from build123d import *

# Parameters (mm, degrees)
SKETCH_1_W               = 145
SKETCH_1_H               = 141.74
EXTRUDE_1_DEPTH          = 1
FILLET_1_R               = 15
EXTRUDE_2_DEPTH          = 1
SKETCH_3_R               = 2.5
SKETCH_3_R_2             = 1.5
CUT_EXTRUDE_1_DEPTH      = 127.962285976
PATTERN_CIRCULAR_1_COUNT = 4
CUT_EXTRUDE_2_DEPTH      = 127.962285976
FILLET_2_R               = 15
FILLET_3_R               = 3
CUT_EXTRUDE_3_DEPTH      = 121.297119251
SKETCH_6_W               = 36
SKETCH_6_H               = 1
EXTRUDE_3_DEPTH          = 6
FILLET_4_R               = 10
FILLET_5_R               = 1.5
SKETCH_8_W               = 20
SKETCH_8_H               = 8
SKETCH_8_R               = 1.5
EXTRUDE_5_DEPTH          = 1
FILLET_8_R               = 3
FILLET_9_R               = 5


with BuildPart() as part:
    # 草图1 → 凸台-拉伸1 (new body)
    with BuildSketch(Plane(origin=(0, 0, 0), x_dir=(1, 0, 0), z_dir=(0, 1, 0))):
        Rectangle(SKETCH_1_W, SKETCH_1_H)
    extrude(amount=EXTRUDE_1_DEPTH)

    # 圆角1
    fillet_1_edges = [part.edges().sort_by_distance(p)[0] for p in [
        (-72.5, 0.5, -70.87),
    ]]
    fillet(fillet_1_edges, radius=FILLET_1_R)

    # 草图2 → 凸台-拉伸2 (add)
    with BuildSketch(Plane(origin=(0, 1, 0), x_dir=(1, 0, 0), z_dir=(0, 1, 0))):
        with BuildLine():
            Line((-92.747934341, -37.981190359), (-72.5, -22.981190359))
            Line((-72.5, -22.981190359), (-72.5, -81.673631364))
            Line((-72.5, -81.673631364), (-94.803937304, -53.673631364))
            ThreePointArc((-94.803937304, -53.673631364), (-97.10678595, -45.391007263), (-92.747934341, -37.981190359))
        make_face()
    extrude(amount=-EXTRUDE_2_DEPTH)

    # 草图3 → 切除-拉伸1 (cut, through all)
    with BuildSketch(Plane(origin=(0, 1, 0), x_dir=(1, 0, 0), z_dir=(0, 1, 0))):
        with Locations(Location((-86.2, -46.82, 0), (0, 0, 270))):
            Circle(SKETCH_3_R)
        with Locations(Location((-93.2, -46.82, 0), (0, 0, 270))):
            Circle(SKETCH_3_R_2)
    cut_extrude_1 = extrude(amount=-CUT_EXTRUDE_1_DEPTH, mode=Mode.SUBTRACT)

    # 阵列(圆周)1: 切除-拉伸1 ×4 about axis
    pattern_circular_1_axis = Axis((-86.2, 0, 46.82), (0, 1, 0))
    for i in range(1, PATTERN_CIRCULAR_1_COUNT):
        add(cut_extrude_1.rotate(pattern_circular_1_axis, i * 360 / PATTERN_CIRCULAR_1_COUNT), mode=Mode.SUBTRACT)

    # 草图4 → 切除-拉伸2 (cut, through all)
    with BuildSketch(Plane(origin=(0, 1, 0), x_dir=(1, 0, 0), z_dir=(0, 1, 0))):
        Polygon((-72.5, -70.87), (-94.803937304, -53.673631364), (-72.5, -88.862813476), align=None)
    extrude(amount=-CUT_EXTRUDE_2_DEPTH, mode=Mode.SUBTRACT)

    # 圆角2
    fillet_2_edges = [part.edges().sort_by_distance(p)[0] for p in [
        (-72.5, 0.5, 70.87),
    ]]
    fillet(fillet_2_edges, radius=FILLET_2_R)

    # 圆角3
    fillet_3_edges = [part.edges().sort_by_distance(p)[0] for p in [
        (-72.5, 0.5, 22.981190359),
    ]]
    fillet(fillet_3_edges, radius=FILLET_3_R)

    # 草图5 → 切除-拉伸3 (cut, through all)
    with BuildSketch(Plane(origin=(0, 1, 0), x_dir=(1, 0, 0), z_dir=(0, 1, 0))):
        with BuildLine():
            Line((-50, 60.87), (50, 60.87))
            ThreePointArc((50, 60.87), (58, 52.87), (50, 44.87))
            Line((50, 44.87), (-50, 44.87))
            ThreePointArc((-50, 44.87), (-58, 52.87), (-50, 60.87))
        make_face()
        with BuildLine():
            Line((-50, 39.87), (50, 39.87))
            ThreePointArc((50, 39.87), (58, 31.87), (50, 23.87))
            Line((50, 23.87), (-50, 23.87))
            ThreePointArc((-50, 23.87), (-58, 31.87), (-50, 39.87))
        make_face()
        with BuildLine():
            Line((-50, 18.87), (50, 18.87))
            ThreePointArc((50, 18.87), (58, 10.87), (50, 2.87))
            Line((50, 2.87), (-50, 2.87))
            ThreePointArc((-50, 2.87), (-58, 10.87), (-50, 18.87))
        make_face()
        with BuildLine():
            Line((-50, -2.13), (50, -2.13))
            ThreePointArc((50, -2.13), (58, -10.13), (50, -18.13))
            Line((50, -18.13), (-50, -18.13))
            ThreePointArc((-50, -18.13), (-58, -10.13), (-50, -2.13))
        make_face()
        with BuildLine():
            Line((-50, -23.13), (50, -23.13))
            ThreePointArc((50, -23.13), (58, -31.13), (50, -39.13))
            Line((50, -39.13), (-50, -39.13))
            ThreePointArc((-50, -39.13), (-58, -31.13), (-50, -23.13))
        make_face()
        with BuildLine():
            Line((-50, -44.13), (50, -44.13))
            ThreePointArc((50, -44.13), (58, -52.13), (50, -60.13))
            Line((50, -60.13), (-50, -60.13))
            ThreePointArc((-50, -60.13), (-58, -52.13), (-50, -44.13))
        make_face()
    extrude(amount=-CUT_EXTRUDE_3_DEPTH, mode=Mode.SUBTRACT)

    # 草图6 → 凸台-拉伸3 (add)
    with BuildSketch(Plane(origin=(0, 0, -70.87), x_dir=(-1, 0, 0), z_dir=(0, 0, -1))):
        with Locations((-54.5, 0.5)):
            Rectangle(SKETCH_6_W, SKETCH_6_H)
    extrude(amount=EXTRUDE_3_DEPTH)

    # 圆角4
    fillet_4_edges = [part.edges().sort_by_distance(p)[0] for p in [
        (72.5, 0.5, -76.87),
    ]]
    fillet(fillet_4_edges, radius=FILLET_4_R)

    # 圆角5
    fillet_5_edges = [part.edges().sort_by_distance(p)[0] for p in [
        (36.5, 0.5, -76.87),
    ]]
    fillet(fillet_5_edges, radius=FILLET_5_R)

    # 草图8 → 凸台-拉伸5 (add)
    with BuildSketch(Plane(origin=(0, 1, 0), x_dir=(1, 0, 0), z_dir=(0, 1, 0))):
        with Locations((52.5, -74.87)):
            Rectangle(SKETCH_8_W, SKETCH_8_H)
        with Locations(Location((47.504832843, -73.37, 0), (0, 0, 270))):
            Circle(SKETCH_8_R, mode=Mode.SUBTRACT)
        with Locations(Location((57.504832843, -73.37, 0), (0, 0, 270))):
            Circle(SKETCH_8_R, mode=Mode.SUBTRACT)
    extrude(amount=-EXTRUDE_5_DEPTH)

    # 圆角8
    fillet_8_edges = [part.edges().sort_by_distance(p)[0] for p in [
        (62.5, 0.5, 70.87),
        (62.5, 0.5, 78.87),
        (42.5, 0.5, 78.87),
        (42.5, 0.5, 70.87),
    ]]
    fillet(fillet_8_edges, radius=FILLET_8_R)

    # 圆角9
    fillet_9_edges = [part.edges().sort_by_distance(p)[0] for p in [
        (72.5, 0.5, 70.87),
    ]]
    fillet(fillet_9_edges, radius=FILLET_9_R)


solid = part.part
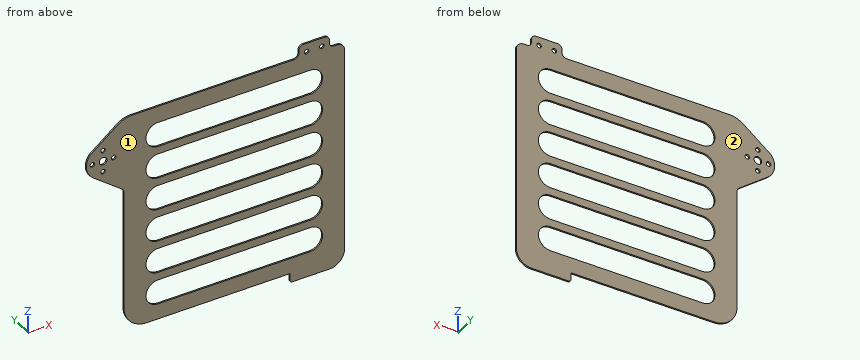
Verification items for the finished model (mm, model axes). Face numbers are marked on the shaded views. Coordinates: 2 decimals unless noted, no trailing zeros. Order: outer loops, then holes, each group sorted by start corner. A loop starts at its lowest first (then second) coordinate and runs counter-clockwise, first axis right, second up.
Item 1: Section check C-C, the plane y = 0.65. Give the number of separate pieces and of enclosed holes in the cut face, then the cut area to 3 significant figures.
Filled in:
separate pieces: 1
enclosed holes: 13
area: 10,700 mm2
Item 2: Depth check by flat-ended pin: pin 1 (6 mm diameter, centred on x = -62.5, z = 62.5, fed in from -Y); pin 2 (0.5 mm diameter, centred on x = 6.5, y = 0.5, fed in from -Z); pin 3 (4.5 mm diameter, centred on x = -86.2, z = 46.82, fed in from +Y); pin 4 (0.5 mm diameter, centred on x = 3, y = 0.5, fed in from +Z). Enter the tip coordinate at first touch or a pass-through.
Filled in:
pin 1: stops at y = 0
pin 2: stops at z = -70.87
pin 3: passes through
pin 4: stops at z = 70.87
Item 3: Section check A-A, the plane z = -52.87. Enter the section's corners in (x, y), then the cut area to 3 significant figures.
Filled in:
outline: (-72.5, 0) - (-58, 0) - (-58, 1) - (-72.5, 1) - close; (58, 0) - (72.5, 0) - (72.5, 1) - (58, 1) - close
area: 29.0 mm2
Item 4: Release check for a two-part mould opening along Y. For the marked faces 1 and 2 record: +Y half, -Y half, draft (parallel to the pull), parting line (faces both ways), or undercut.
Filled in:
face 1: -Y half
face 2: +Y half
Item 5: Material ranges on L1, parallel to X at y = 0.6, z = 73.37; L2, parallel to X at y = 0.35, z = 53.82; L3, parallel to X at y = 0.8, z = 46, recorded low to high.
Filled in:
L1: x = 42.46 to 46, 49 to 56, 59 to 62.54
L2: x = -94.61 to -87.7, -84.7 to -57.82, 57.82 to 72.5
L3: x = -97.17 to -94.46, -91.94 to -88.56, -83.84 to -80.46, -77.94 to -55.14, 55.14 to 72.5
Item 6: Section check B-B, the plane x = -65. Enter the section's corners in (y, z), then the cut area to 3 significant figures.
Filled in:
outline: (0, -68.86) - (1, -68.86) - (1, 70.87) - (0, 70.87) - close
area: 140 mm2
